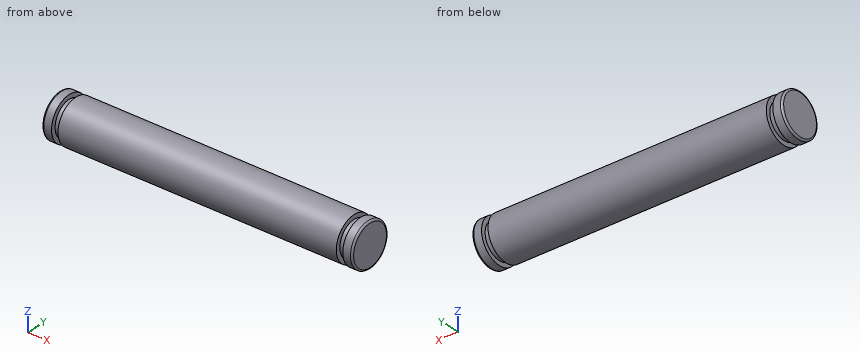
from build123d import *


with BuildPart() as part:
    # Sketch1 → Revolve1 (revolve)
    with BuildSketch(Plane(origin=(0, 0, 0), x_dir=(1, 0, 0), z_dir=(0, 1, 0))):
        with BuildLine():
            Line((-15.927, 2.5), (15.927, 2.5))
            Line((15.927, 2.5), (15.927, 2))
            Line((15.927, 2), (16.667, 2))
            Line((16.667, 2), (16.667, 2.5))
            Line((16.667, 2.5), (17.55, 2.5))
            ThreePointArc((17.55, 2.5), (17.691421356, 2.441421356), (17.75, 2.3))
            Line((17.75, 2.3), (17.75, 0))
            Line((17.75, 0), (-17.75, 0))
            Line((-17.75, 0), (-17.75, 2.3))
            ThreePointArc((-17.75, 2.3), (-17.691421356, 2.441421356), (-17.55, 2.5))
            Line((-17.55, 2.5), (-16.667, 2.5))
            Line((-16.667, 2.5), (-16.667, 2))
            Line((-16.667, 2), (-15.927, 2))
            Line((-15.927, 2), (-15.927, 2.5))
        make_face()
    revolve(axis=Axis((17.75, 0, 0), (-1, 0, 0)))


solid = part.part
For this review, take the finished solid that the model builds, in its own axes (mm). Round coordinates to 2 decimals unless told otherwise and drop trailing zeros. Order: outer loops, then holes, each group sorted by start corner. A loop starts at its lowest first (then second) coordinate and runs counter-clockwise, first axis right, second up. Notation, with made-up numbers: (0.25, 50.5) -> (50.25, 50.5) arc R15 cw to (50.25, 58.5) -> close; hole circle Ø4 at (75.25, -9.5). An arc over 180 degrees is marked (long way). Put each result on its own line as item: value.
Q1. Add section A-A on x = -2.5. Write out the cut boundary in (y, z), plus the area to 3 significant figures.
Check result:
outline: circle Ø5 at (0, 0)
area: 19.6 mm2
Q2. For probe 1 along X at (y, z) = (-1.6, 1.4); probe 2 along Y at (x, z) = (-14, -1.75), list the stretches that pass through material, from the lowest coordinate up. Write a range as [from, to].
Check result:
probe 1: [-17.75, -16.67], [-15.93, 15.93], [16.67, 17.75]
probe 2: [-1.79, 1.79]
Q3. Insertion check: pin 1 Ø2 at (x, z) = (4.5, 1.5) entering from -Y. The pin has a flat end and moves straight along its axis. Give the tip position at first contact, or say it passes through.
Check result:
pin 1: y = -2.45
